For this review, take the finished solid that the model builds, in its own axes (mm). A direction names the side the tool comes from. Round coordinates to 2 decimals unless told otherwise and drop trailing zeros. Order: outer loops, then holes, each group sorted by start corner. A loop starts at its lowest first (then second) coordinate and runs counter-clockwise, first axis right, second up. Notation, with made-up numbers: M 77.5,31.5 L 95.5,31.5 A36 ccw 95.5,67.5 Z; hole C 54,-17.75 d10. An arc over 180 degrees is marked long. Answer as a JSON object with one key per item and string values.
from build123d import *

# Parameters (mm, degrees)
SKETCH1_R           = 1.6
BOSS_EXTRUDE1_DEPTH = 3.4
SKETCH2_R           = 1.6
BOSS_EXTRUDE2_DEPTH = 1.7
SKETCH3_W           = 20.1
SKETCH3_H           = 3
CUT_EXTRUDE1_DEPTH  = 1.7


with BuildPart() as part:
    # Sketch1 → Boss-Extrude1 (new body)
    with BuildSketch(Plane(origin=(0, 80.955025863, 0), x_dir=(1, 0, 0), z_dir=(0, 1, 0))):
        with BuildLine():
            Line((86.165130669, -156.732155685), (116.645130669, -156.732155685))
            ThreePointArc((116.645130669, -156.732155685), (118.441181893, -157.47610446), (119.185130669, -159.272155685))
            Line((119.185130669, -159.272155685), (119.185130669, -169.432155685))
            Line((119.185130669, -169.432155685), (83.625130669, -169.432155685))
            Line((83.625130669, -169.432155685), (83.625130669, -159.272155685))
            ThreePointArc((83.625130669, -159.272155685), (84.369079444, -157.47610446), (86.165130669, -156.732155685))
        make_face()
        with Locations(Location((116.03690482, -166.898975693, 0), (0, 0, 270))):
            Circle(SKETCH1_R, mode=Mode.SUBTRACT)
        with Locations(Location((112.914749612, -160.090079663, 0), (0, 0, 270))):
            Circle(SKETCH1_R, mode=Mode.SUBTRACT)
        with Locations(Location((89.895511725, -160.090079663, 0), (0, 0, 270))):
            Circle(SKETCH1_R, mode=Mode.SUBTRACT)
        with Locations(Location((86.773356517, -166.898975693, 0), (0, 0, 270))):
            Circle(SKETCH1_R, mode=Mode.SUBTRACT)
    extrude(amount=BOSS_EXTRUDE1_DEPTH)

    # Sketch2 → Boss-Extrude2 (add)
    # profile 1 of 2: a face of its own
    with BuildSketch(Plane(origin=(0, 84.355025863, 0), x_dir=(1, 0, 0), z_dir=(0, 1, 0))):
        with BuildLine():
            Line((83.625130669, -169.432155685), (91.355130669, -169.432155685))
            Line((91.355130669, -169.432155685), (91.355130669, -176.877155685))
            ThreePointArc((91.355130669, -176.877155685), (90.611181893, -178.673206909), (88.815130669, -179.417155685))
            Line((88.815130669, -179.417155685), (86.165130669, -179.417155685))
            ThreePointArc((86.165130669, -179.417155685), (84.369079444, -178.673206909), (83.625130669, -176.877155685))
            Line((83.625130669, -176.877155685), (83.625130669, -169.432155685))
        make_face()
        with Locations(Location((88.655130669, -175.867155685, 0), (0, 0, 270))):
            Circle(SKETCH2_R, mode=Mode.SUBTRACT)
    # profile 2 of 2: a face of its own
    with BuildSketch(Plane(origin=(0, 84.355025863, 0), x_dir=(1, 0, 0), z_dir=(0, 1, 0))):
        with BuildLine():
            Line((119.185130669, -169.432155685), (111.455130669, -169.432155685))
            Line((111.455130669, -169.432155685), (111.455130669, -176.877155685))
            ThreePointArc((111.455130669, -176.877155685), (112.199079444, -178.673206909), (113.995130669, -179.417155685))
            Line((113.995130669, -179.417155685), (116.645130669, -179.417155685))
            ThreePointArc((116.645130669, -179.417155685), (118.441181893, -178.673206909), (119.185130669, -176.877155685))
            Line((119.185130669, -176.877155685), (119.185130669, -169.432155685))
        make_face()
        with Locations(Location((114.155130669, -175.867155685, 0), (0, 0, 270))):
            Circle(SKETCH2_R, mode=Mode.SUBTRACT)
    extrude(amount=-BOSS_EXTRUDE2_DEPTH)

    # Sketch3 → Cut-Extrude1 (cut)
    with BuildSketch(Plane(origin=(0, 84.355025863, 0), x_dir=(1, 0, 0), z_dir=(0, 1, 0))):
        with Locations((101.405130669, -167.932155685)):
            Rectangle(SKETCH3_W, SKETCH3_H)
    extrude(amount=-CUT_EXTRUDE1_DEPTH, mode=Mode.SUBTRACT)


solid = part.part
1) Insertion check: P1, Ø3.5, axis at x = 102.5, z = 168.5, coming from the +Y side (3 decimals); P2, Ø0.5, axis at x = 98.5, y = 84, coming from the +Z side; P3, Ø4, axis at x = 114.16, z = 175.87, coming from the -Y side (3 decimals). Each pin has a flat end and moves straight along its axis. Give the tip position at first contact, or say it passes through.
Geometry check:
{"P1": "stops at y = 82.655", "P2": "stops at z = 166.43", "P3": "stops at y = 82.655"}
2) Add section C-C on z = 174.75. State the section outline as (x, y) points, and give its area (3 significant figures).
Geometry check:
{"outline": "M 83.63,82.66 L 87.51,82.66 L 87.51,84.36 L 83.63,84.36 Z; M 89.8,82.66 L 91.36,82.66 L 91.36,84.36 L 89.8,84.36 Z; M 111.46,82.66 L 113.01,82.66 L 113.01,84.36 L 111.46,84.36 Z; M 115.3,82.66 L 119.19,82.66 L 119.19,84.36 L 115.3,84.36 Z", "area": "18.5 mm²"}
3) Add section A-A on z = 170.25. State the section outline as (x, y) points, and give its area (3 significant figures).
Geometry check:
{"outline": "M 83.63,82.66 L 91.36,82.66 L 91.36,84.36 L 83.63,84.36 Z; M 111.46,82.66 L 119.19,82.66 L 119.19,84.36 L 111.46,84.36 Z", "area": "26.3 mm²"}
4) For L1, parallel to X at y = 82.7, z = 170.25; L2, parallel to X at y = 82.95, z = 159.5; L3, parallel to X at y = 81.8, z = 165.5, list the stretches that pass through material, from the lowest coordinate up.
Geometry check:
{"L1": "x = 83.63 to 91.36, 111.46 to 119.19", "L2": "x = 83.63 to 88.41, 91.38 to 111.43, 114.4 to 119.19", "L3": "x = 83.63 to 86, 87.55 to 115.26, 116.81 to 119.19"}
5) Add section B-B on x = 113.5. State the section outline as (y, z) points, and give its area (3 significant figures).
Geometry check:
{"outline": "M 80.96,156.73 L 84.36,156.73 L 84.36,158.6 L 80.96,158.6 Z; M 80.96,161.58 L 84.36,161.58 L 84.36,174.41 L 82.66,174.41 L 82.66,169.43 L 80.96,169.43 Z; M 82.66,177.33 L 84.36,177.33 L 84.36,179.37 L 82.66,179.37 Z", "area": "45.0 mm²"}
6) Machinability: for faces 1 (the cylindrical face through (84.349, 82.631, 157.496)), 2 (the cylindrical face through (90.977, 82.631, 158.911)), 3 (the flat face through (101, 82.655, 168)), 4 (the flat face through (88, 82.655, 174)), 5 (the cylindrical face through (112.179, 83.517, 178.653)), which of the approach directions +Z, -Z, +X, -X, +Y, -Y give a long, thin tool a straight path to every point of the face, cutting with its end or side? Answer none if there is none.
Geometry check:
{"face 1": "-Z, -X, +Y, -Y", "face 2": "+Y, -Y", "face 3": "+Z, +Y", "face 4": "+Z, +X, -X, -Y", "face 5": "+Z, +Y, -Y"}
7) Add section D-D on y = 81.55. State the section outline as (x, z) points.
Geometry check:
{"outline": "M 83.63,159.27 A2.54 ccw 86.17,156.73 L 116.65,156.73 A2.54 ccw 119.19,159.27 L 119.19,169.43 L 83.63,169.43 Z; hole C 86.77,166.9 d3.2; hole C 89.9,160.09 d3.2; hole C 112.91,160.09 d3.2; hole C 116.04,166.9 d3.2"}
